Could you check a few things on this drawing? It's one solid part, dimensions in mm from its lowest x, y, z. A direction names the side the tool comes from. Coordinates: 2 decimals unless noted, no trailing zeros. Loops run counter-clockwise (first coordinate to the right, second up) from the corner with the lowest first, then second, coordinate; pieces in that order, holes last. Notation, with made-up numbers: M 1,-24 L 56,-24 A9 cw 56,-12 Z; hole C -11,53 d8. An arc over 180 degrees is marked long. Use one line per item in the form item = value. Start each with the question number.
(1) Imagine slicing it at B-B, the plane z = 14.5. Please give me the cut outline in (x, y).
(2) Please list where these lines run through material, in increasing order: L1, parallel to X at y = 45.5, z = 16; L2, parallel to Y at x = 176.5, z = 4.
(3) Will this pin go through, and if not, where does the flat tip stop? P1, Ø5, axis at x = 259.5, z = 28, coming from the +Y side.
(4) Imagine slicing it at C-C, the plane x = 400. Please give me the cut outline in (y, z), and give its area (3 significant figures).
(5) Thinking about a two-plate mould opening in X: for the marked faces 1, 2 and 3, which applies, +X half, -X half, draft (parallel to the pull), parting line (faces both ways), or undercut?
(6) On a 3-axis mill with a long thin cutter (end or side, diameter ignored), from which of +Z, -Z, +X, -X, +Y, -Y can I reach the whole of each face in a straight line? I mean the marked faces 4 and 5. Say none if no direction works.
(7) Imagine slicing it at A-A, the plane y = 51. Please give me the cut outline in (x, z).
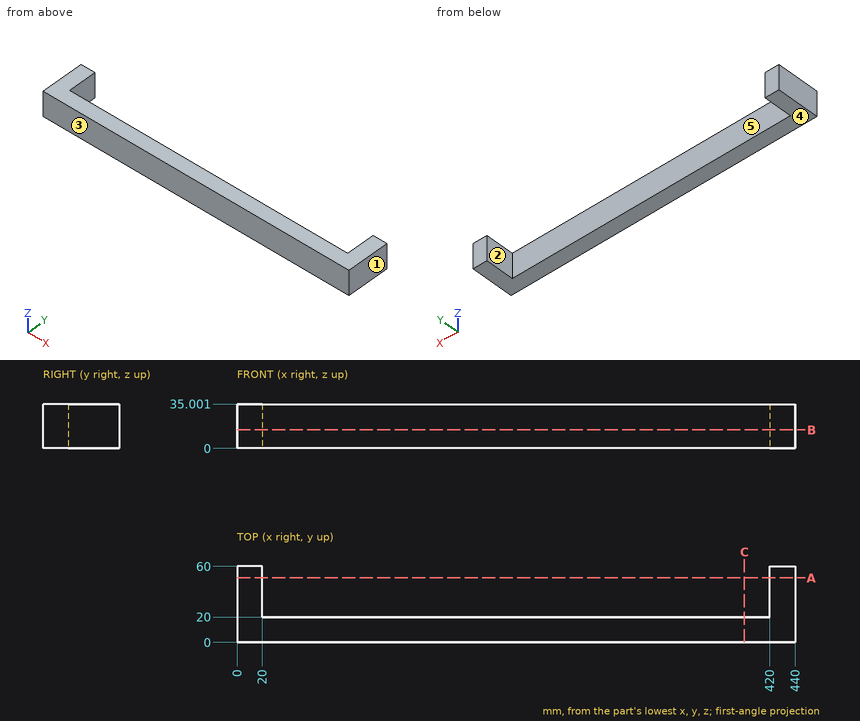
Answer:
q1.outline = M 0,0 L 440,0 L 440,60 L 420,60 L 420,20 L 20,20 L 20,60 L 0,60 Z
q2.L1 = 0 to 20, 420 to 440
q2.L2 = 0 to 20
q3.P1 = 20
q4.outline = M 0,0 L 20,0 L 20,35 L 0,35 Z
q4.area = 700 mm²
q5.face_1 = +X half
q5.face_2 = undercut
q5.face_3 = draft
q6.face_4 = -Z, +X, -X, +Y, -Y
q6.face_5 = +Z, -Z, +Y
q7.outline = M 0,0 L 20,0 L 20,35 L 0,35 Z; M 420,0 L 440,0 L 440,35 L 420,35 Z
